The model under review builds one solid part; all positions refer to its coordinate system, in mm. Round coordinates to 2 decimals unless told otherwise and drop trailing zeros. Loops run counter-clockwise (first coordinate to the right, second up) from the corner with the lowest first, then second, coordinate; pieces in that order, holes last. Notation, with made-up numbers: M 13,84 L 48,84 A23 cw 48,114 Z; hole C -0.5,55.25 d5. An arc over 180 degrees is marked long. Answer as a JSON object with one key per item and string values. Group by question number.
Item 1: Consider section B-B (x = 242.5). Give the boundary of the cut face in (y, z), and give its area (3 significant figures).
Item 2: Insertion check: P1, Ø8, axis at x = 453, y = -3.5, coming from the +Z side; P2, Ø6, axis at y = -5, z = -185, coming from the -X side. Each pin has a flat end and moves straight along its axis. Give the tip position at first contact, or say it passes through.
Item 3: Consider section A-A (z = -181). Give the boundary of the cut face in (x, y).
Item 4: To check wall thickness, follow line 1 (Y direction, x = 90, z = -173.75); line 2 (Z direction, x = 248.5, y = 2); line 3 (Z direction, x = 552.5, y = -9). State the ranges of each line that lie inside material, in increasing order.
```python
from build123d import *

# Parameters (mm, degrees)
BOSS_EXTRUDE1_START = 30
BOSS_EXTRUDE1_DEPTH = 572


with BuildPart() as part:
    # Sketch4 → Boss-Extrude1 (new body)
    with BuildSketch(Plane(origin=(0, 0, 0), x_dir=(0, 0, -1), z_dir=(1, 0, 0)).offset(BOSS_EXTRUDE1_START)):
        with BuildLine():
            Line((195, 13), (195, -13))
            ThreePointArc((195, -13), (194.414213562, -14.414213562), (193, -15))
            Line((193, -15), (168, -15))
            ThreePointArc((168, -15), (166.585786438, -14.414213562), (166, -13))
            Line((166, -13), (166, -12))
            ThreePointArc((166, -12), (166.585786438, -10.585786438), (168, -10))
            Line((168, -10), (188, -10))
            ThreePointArc((188, -10), (189.414213562, -9.414213562), (190, -8))
            Line((190, -8), (190, 8))
            ThreePointArc((190, 8), (189.414213562, 9.414213562), (188, 10))
            Line((188, 10), (168, 10))
            ThreePointArc((168, 10), (166.585786438, 10.585786438), (166, 12))
            Line((166, 12), (166, 13))
            ThreePointArc((166, 13), (166.585786438, 14.414213562), (168, 15))
            Line((168, 15), (193, 15))
            ThreePointArc((193, 15), (194.414213562, 14.414213562), (195, 13))
        make_face()
    extrude(amount=BOSS_EXTRUDE1_DEPTH)


solid = part.part
```
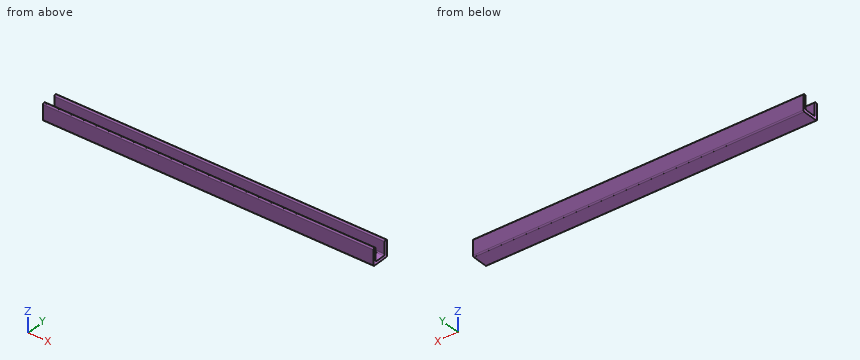
Geometry results:
{
 "1": {"outline": "M -15,-193 A2 ccw -13,-195 L 13,-195 A2 ccw 15,-193 L 15,-168 A2 ccw 13,-166 L 12,-166 A2 ccw 10,-168 L 10,-188 A2 cw 8,-190 L -8,-190 A2 cw -10,-188 L -10,-168 A2 ccw -12,-166 L -13,-166 A2 ccw -15,-168 Z", "area": "387 mm^2"},
 "2": {"P1": "stops at z = -190", "P2": "passes through"},
 "3": {"outline": "M 30,-15 L 602,-15 L 602,-10 L 30,-10 Z; M 30,10 L 602,10 L 602,15 L 30,15 Z"},
 "4": {"line 1": "y = -15 to -10, 10 to 15", "line 2": "z = -195 to -190", "line 3": "z = -195 to -189.73"}
}
